Check sheet for the modelled part. Datum: model origin and axes. Units: mm. Face numbers are marked on the shaded views. A direction names the side the tool comes from. Round coordinates to 2 decimals unless told otherwise and drop trailing zeros. Loops run counter-clockwise (first coordinate to the right, second up) from the corner with the lowest first, then second, coordinate; pieces in that order, holes last. Notation, with made-up numbers: (6, 63) - (30, 63) arc R21 ccw to (30, 75) - close; hole circle Ø2 at (31.25, 1.25). An arc over 180 degrees is marked (long way). Return JSON: item names as keys, results as strings.
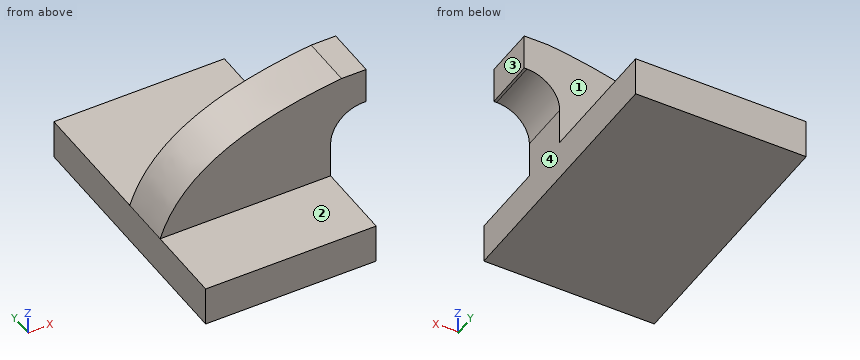
from build123d import *

# Parameters (mm, degrees)
F1_DEPTH = 63.5
F2_DEPTH = 25.4


with BuildPart() as f1:
    # F0 (on Front) → F1 (new body, symmetric)
    with BuildSketch(Plane.XZ):
        Polygon((-41.275, -9.525), (41.275, -9.525), (41.275, 9.525), (22.225, 9.525), (-41.275, 9.525), align=None)
    extrude(amount=F1_DEPTH, both=True)

    # F0 (on Front) → F2 (join)
    with BuildSketch(Plane.XZ):
        with BuildLine():
            Line((22.225, 9.525), (41.275, 9.525))
            Line((41.275, 9.525), (41.275, 27.0002))
            ThreePointArc((41.275, 27.0002), (45.92468, 38.22552), (57.15, 42.8752))
            Line((57.15, 42.8752), (58.455468, 42.8752))
            Line((58.455468, 42.8752), (58.455468, 60.276241))
            Line((58.455468, 60.276241), (46.545251, 60.276241))
            ThreePointArc((46.545251, 60.276241), (28.953134, 47.608266), (22.225, 27.0002))
            Line((22.225, 27.0002), (22.225, 9.525))
        make_face()
        with BuildLine():
            add(Edge.make_bspline(
                [(-41.275, 9.525), (-29.582771, 44.333433), (8.860969, 55.563996), (46.545251, 60.276241)],
                knots=[0, 0, 0, 0, 101.430197, 101.430197, 101.430197, 101.430197], degree=3))
            Line((-41.275, 9.525), (22.225, 9.525))
            Line((22.225, 9.525), (22.225, 27.0002))
            ThreePointArc((22.225, 27.0002), (28.953134, 47.608266), (46.545251, 60.276241))
        make_face()
    extrude(amount=F2_DEPTH)


solid = f1.part
Q1. Sectioned sample at A-A (y = -29.5). Enter the section's corners in (x, z) (3 decimals), plus the area to 3 significant figures.
Answer key:
{"outline": "(-41.275, -9.525) - (41.275, -9.525) - (41.275, 9.525) - (-41.275, 9.525) - close", "area": "1,570 mm²"}
Q2. Depth check by flat-ended pin: P1, Ø10, axis at x = 10, z = 16, coming from the +Y side; P2, Ø2, axis at y = 15, z = 3.5, coming from the +X side (3 decimals); P3, Ø1, axis at x = 21, y = 23.5, coming from the +Z side (3 decimals). Enter the tip coordinate at first touch or a pass-through.
Answer key:
{"P1": "stops at y = 0", "P2": "stops at x = 41.275", "P3": "stops at z = 9.525"}
Q3. Scan lines: probe 1 along Y at (x, z) = (6, 31); probe 2 along X at (y, z) = (48.5, 5.5) (3 decimals); probe 3 along Z at (x, y) = (25.5, -47) (3 decimals). Record each from-to range of solid material in increasing order. Write a range as [from, to].
Answer key:
{"probe 1": "y = [-25.4, 0]", "probe 2": "x = [-41.275, 41.275]", "probe 3": "z = [-9.525, 9.525]"}
Q4. Tool access check on the marked faces 1, 2, 3 and 4. Record the directions out of +Z, -Z, +X, -X, +Y, -Y that give a thin tool (end or side, any length) a straight path to the whole face; none if there is none.
Answer key:
{"face 1": "+Z, +X, -X, +Y", "face 2": "+Z, +X, -X, -Y", "face 3": "+Z, -Z, +X, +Y, -Y", "face 4": "-Z, +X, +Y, -Y"}
Q5. Sectioned sample at B-B (x = 48.5). Enter the section's corners in (y, z).
Answer key:
{"outline": "(-25.4, 40.31) - (0, 40.31) - (0, 60.28) - (-25.4, 60.28) - close"}
